```python
from build123d import *

# Parameters (mm, degrees)
SKETCH2_R           = 2.25
SKETCH2_R_2         = 13
BOSS_EXTRUDE1_DEPTH = 3
BOSS_EXTRUDE2_DEPTH = 50


with BuildPart() as part:
    # Sketch2 → Boss-Extrude1 (new body)
    with BuildSketch(Plane(origin=(0, 0, 0), x_dir=(1, 0, 0), z_dir=(0, 1, 0))):
        with BuildLine():
            Line((85, 0), (85, 103.666002653))
            Line((85, 103.666002653), (15, 103.666002653))
            Line((15, 103.666002653), (15, 83.666002653))
            ThreePointArc((15, 83.666002653), (-65.192024052, -54.543560573), (85, 0))
        make_face()
        with Locations((20.5, 0)):
            Circle(SKETCH2_R, mode=Mode.SUBTRACT)
        with Locations((-20.5, 0)):
            Circle(SKETCH2_R, mode=Mode.SUBTRACT)
        Circle(SKETCH2_R_2, mode=Mode.SUBTRACT)
    extrude(amount=BOSS_EXTRUDE1_DEPTH)

    # Sketch3 → Boss-Extrude2 (add)
    with BuildSketch(Plane(origin=(0, 3, 0), x_dir=(1, 0, 0), z_dir=(0, 1, 0))):
        with BuildLine():
            Line((15, 103.666002653), (18, 103.666002653))
            Line((18, 103.666002653), (18, 80))
            ThreePointArc((18, 80), (-64.031242374, -51.224993899), (82, 0))
            Line((82, 0), (82, 103.666002653))
            Line((82, 103.666002653), (85, 103.666002653))
            Line((85, 103.666002653), (85, 0))
            ThreePointArc((85, 0), (-65.192024052, -54.543560573), (15, 83.666002653))
            Line((15, 83.666002653), (15, 103.666002653))
        make_face()
    extrude(amount=BOSS_EXTRUDE2_DEPTH)


solid = part.part
```
Geometry check sheet. Reference: the model listing, model coordinates, mm. A direction names the side the tool comes from. Coordinates: 2 decimals unless noted, no trailing zeros. Order: outer loops, then holes, each group sorted by start corner. A loop starts at its lowest first (then second) coordinate and runs counter-clockwise, first axis right, second up.
Item 1: Tool access check on faces 4 (the cylindrical face through (22.646, 1.479, -0.676)), 5 (the flat face through (82, 28, -51)). Record the directions out of +Z, -Z, +X, -X, +Y, -Y that give a thin tool (end or side, any length) a straight path to the whole face; none if there is none.
Item 2: Section check C-C (x = 54). Enter the section's corners in (y, z).
Item 3: Section check D-D (z = 22.5). Enter the section's corners in (x, y).
Item 4: Depth check by flat-ended pin: pin 1 (22 mm diameter, centred on y = 22.5, z = -97, fed in from -X); pin 2 (15 mm diameter, centred on y = 30.5, z = -63, fed in from -X); pin 3 (21 mm diameter, centred on x = 0, z = 0, fed in from +Y); pin 4 (5 mm diameter, centred on x = 49.5, y = 11.5, fed in from -Z). Enter the tip coordinate at first touch or a pass-through.
Item 5: Section check A-A (y = 31.5). Enter the section's corners in (x, z).
Item 6: Scan lines: line 1 along Z through (x, y) = (-1, 15); line 2 along X through (y, z) = (12, 2); line 3 along Y through (x, z) = (-28.5, 2). Record each from-to range of solid material in increasing order.
Item 7: Mould release check, pull along Z, two halves, no side actions. Record for faces 1 (the flat face through (47.2, 2.8, -103.666)), 2 (the cylindrical face through (-65.762, 27.65, 48.984)), 3 (the flat face through (15, 26, -94)): released by +Z, released by -Z, zero draft, split by the parting line, or undercut.
Item 8: Section check B-B (x = -20.5). Enter the section's corners in (y, z).
Check sheet entries:
1. face 4: +Y, -Y
1. face 5: -Z, +Y
2. outline: (0, -103.67) - (3, -103.67) - (3, 61.71) - (53, 61.71) - (53, 65.64) - (0, 65.64) - close
3. outline: (-81.97, 0) - (81.97, 0) - (81.97, 53) - (78.85, 53) - (78.85, 3) - (-78.85, 3) - (-78.85, 53) - (-81.97, 53) - close
4. pin 1: stops at x = 15
4. pin 2: stops at x = -64.38
4. pin 3: passes through
4. pin 4: stops at z = 63.4
5. outline: (15, -103.67) - (18, -103.67) - (18, -80) arc R82 cw (long way) to (82, 0) - (82, -103.67) - (85, -103.67) - (85, 0) arc R85 ccw (long way) to (15, -83.67) - close
6. line 1: z = -84.99 to -81.99, 81.99 to 84.99
6. line 2: x = -84.98 to -81.98, 81.98 to 84.98
6. line 3: y = 0 to 3
7. face 1: released by -Z
7. face 2: undercut
7. face 3: zero draft
8. outline: (0, -82.49) - (53, -82.49) - (53, -79.4) - (3, -79.4) - (3, -2.25) - (0, -2.25) - close; (0, 2.25) - (3, 2.25) - (3, 79.4) - (53, 79.4) - (53, 82.49) - (0, 82.49) - close
